from build123d import *

# Parameters (mm, degrees)
SKETCH1_R           = 12.5
BOSS_EXTRUDE1_DEPTH = 36
SKETCH2_R           = 3.5
BOSS_EXTRUDE2_DEPTH = 2.5
SKETCH3_R           = 2
BOSS_EXTRUDE3_DEPTH = 9.5
SKETCH4_R           = 1.641182994
SKETCH4_R_2         = 1.5
CUT_EXTRUDE1_DEPTH  = 5


with BuildPart() as part:
    # Sketch1 → Boss-Extrude1 (new body)
    with BuildSketch(Plane.XY):
        with Locations((-10.215967641, 3.575588675)):
            Circle(SKETCH1_R)
    extrude(amount=BOSS_EXTRUDE1_DEPTH)

    # Sketch2 → Boss-Extrude2 (add)
    with BuildSketch(Plane.XY.offset(36)):
        with Locations((-10.215967641, 3.575588675)):
            Circle(SKETCH2_R)
    extrude(amount=BOSS_EXTRUDE2_DEPTH)

    # Sketch3 → Boss-Extrude3 (add)
    with BuildSketch(Plane.XY.offset(38.5)):
        with Locations((-10.215967641, 3.575588675)):
            Circle(SKETCH3_R)
    extrude(amount=BOSS_EXTRUDE3_DEPTH)

    # Sketch4 → Cut-Extrude1 (cut)
    with BuildSketch(Plane.XY.offset(36)):
        with Locations((-11.143331912, 12.024848731)):
            Circle(SKETCH4_R)
        with Locations((-9.283034314, -4.924411325)):
            Circle(SKETCH4_R_2)
    extrude(amount=-CUT_EXTRUDE1_DEPTH, mode=Mode.SUBTRACT)


solid = part.part
Geometry: final body of the model. Coordinates: model frame, mm. A direction names the side the tool comes from. Give positions to 0.01 mm unless a question says otherwise; leave off trailing zeros. Write each loop counter-clockwise with the first axis right and the second up, starting at its lowest first coordinate (ties: lowest second). Pieces come first, ordered by that corner, then holes. Notation, with made-up numbers: (-30.75, -36) -> (-18.75, -36) arc R26 cw to (-18.75, -15) -> close; hole circle Ø7 at (74.5, 5). An arc over 180 degrees is marked (long way). Answer as a JSON object with one key per item and string values.
1. Contact query for flat-ended pins moving along their axis: pin 1 (5 mm diameter, centred on x = -9.28, y = -4.92, fed in from +Z); pin 2 (10 mm diameter, centred on x = -4, y = 8, fed in from -Z); pin 3 (1.5 mm diameter, centred on y = 5, z = 20, fed in from +X); pin 4 (1.5 mm diameter, centred on x = -9, y = -4.5, fed in from +Z). Output: stop coordinate, or through.
Ans:
{"pin 1": "stops at z = 36", "pin 2": "stops at z = 0", "pin 3": "stops at x = 2.27", "pin 4": "stops at z = 31"}
2. Cut plane D-D on y = 5. Output: boundary loops of the cut face in (x, z), and give its area (3 significant figures).
Ans:
{"outline": "(-22.63, 0) -> (2.2, 0) -> (2.2, 36) -> (-7.02, 36) -> (-7.02, 38.5) -> (-8.81, 38.5) -> (-8.81, 48) -> (-11.62, 48) -> (-11.62, 38.5) -> (-13.41, 38.5) -> (-13.41, 36) -> (-22.63, 36) -> close", "area": "937 mm^2"}
3. Mould query, pull axis X, two halves, no side actions, for faces 1 (the cylindrical face through (1.707, 7.33, 17.748)), 2 (the cylindrical face through (-10.26, 13.41, 33.53)), 3 (the flat face through (-10, 1, 38.5)). Classes: pulls with the +X half, pulls with the -X half, needs draft (parallel to the pull), parting line crosses it, or undercut.
Ans:
{"face 1": "parting line crosses it", "face 2": "undercut", "face 3": "needs draft"}
4. Access query for faces 4 (the cylindrical face through (-10.39, -3.91, 33.53)), 5 (the flat face through (-10, 4, 0)). Directions: +Z, -Z, +X, -X, +Y, -Y. A direction counts if a zero-diameter tool reaches every point of the face in a straight line with its end or side. Return the directions, or none.
Ans:
{"face 4": "+Z", "face 5": "-Z, +X, -X, +Y, -Y"}
5. Cut plane C-C on z = 41. Output: boundary loops of the cut face in (x, y).
Ans:
{"outline": "circle Ø4 at (-10.22, 3.58)"}
6. Cut plane B-B on y = -4. Output: boundary loops of the cut face in (x, z), and give its area (3 significant figures).
Ans:
{"outline": "(-20.16, 0) -> (-0.27, 0) -> (-0.27, 36) -> (-8.1, 36) -> (-8.1, 31) -> (-10.46, 31) -> (-10.46, 36) -> (-20.16, 36) -> close", "area": "704 mm^2"}
7. Ray query, probe 1 along Z at (x, y) = (-15.25, 7); probe 2 along Z at (x, y) = (-11.5, 11.75); probe 3 along Y at (x, z) = (0.75, 21.5). Return the intervals inside material, ascending. Write a range as from..to.
Ans:
{"probe 1": "z = 0..36", "probe 2": "z = 0..31", "probe 3": "y = -2.42..9.58"}
8. Cut plane A-A on x = -9. Output: boundary loops of the cut face in (y, z).
Ans:
{"outline": "(-8.87, 0) -> (16.02, 0) -> (16.02, 36) -> (6.86, 36) -> (6.86, 38.5) -> (5.16, 38.5) -> (5.16, 48) -> (1.99, 48) -> (1.99, 38.5) -> (0.29, 38.5) -> (0.29, 36) -> (-3.45, 36) -> (-3.45, 31) -> (-6.4, 31) -> (-6.4, 36) -> (-8.87, 36) -> close"}
